Study the drawing (mm; zero at the part's minimum x, y, z) and answer. A direction names the side the tool comes from. Give positions to 0.01 mm unless a question says otherwise; leave off trailing zeros. Write each loop counter-clockwise with the first axis right and the second up, starting at its lowest first coordinate (ties: lowest second). Pieces come first, ordered by that corner, then holes. Notation, with made-up numbers: M 64.5,46 L 99.5,46 A14 cw 99.5,62 Z; hole C 77.5,31 d1. An arc over 180 degrees is marked long. Use a Markdown table: item, result. Add a question column.
Item 1: For the marked faces 1, 2, 3, 4 and 5, determine the directions among +Z, -Z, +X, -X, +Y, -Y from which every point of the face is accessible in a straight line to the end or side of a thin tool.
Item 2: Given P1, Ø7.5, axis at x = 6.35, y = 6.35, coming from the +Z side; P2, Ø3, axis at x = 7.5, z = 15.5, coming from the +Y side; P3, Ø1.5, axis at y = 4, z = 35.5, coming from the -X side; P4, Ø5, axis at x = 6, z = 9.5, coming from the -Y side, each flat-ended and moving along its own axis, determine where each tip first touches the part or whether it passes through.
Item 3: A cutting plane is placed at C-C on z = 29. Determine the outline of the cut face in (x, y), then the cut area to 3 significant figures.
Item 4: A cutting plane is placed at A-A on y = 6.35. Determine the outline of the cut face in (x, z) (3 decimals).
Item 5: A cutting plane is placed at B-B on x = 6.35. Determine the outline of the cut face in (y, z) (3 decimals), then the cut area to 3 significant figures.
Item 6: Consider probe 1 along Y at (x, z) = (6.35, 3) (3 decimals); probe 2 along X at (y, z) = (6.5, 15.5); probe 3 along Z at (x, y) = (4.75, 6.75) (3 decimals). Determine where each line is inside the solid, lowest interval first. Write a range as [from, to].
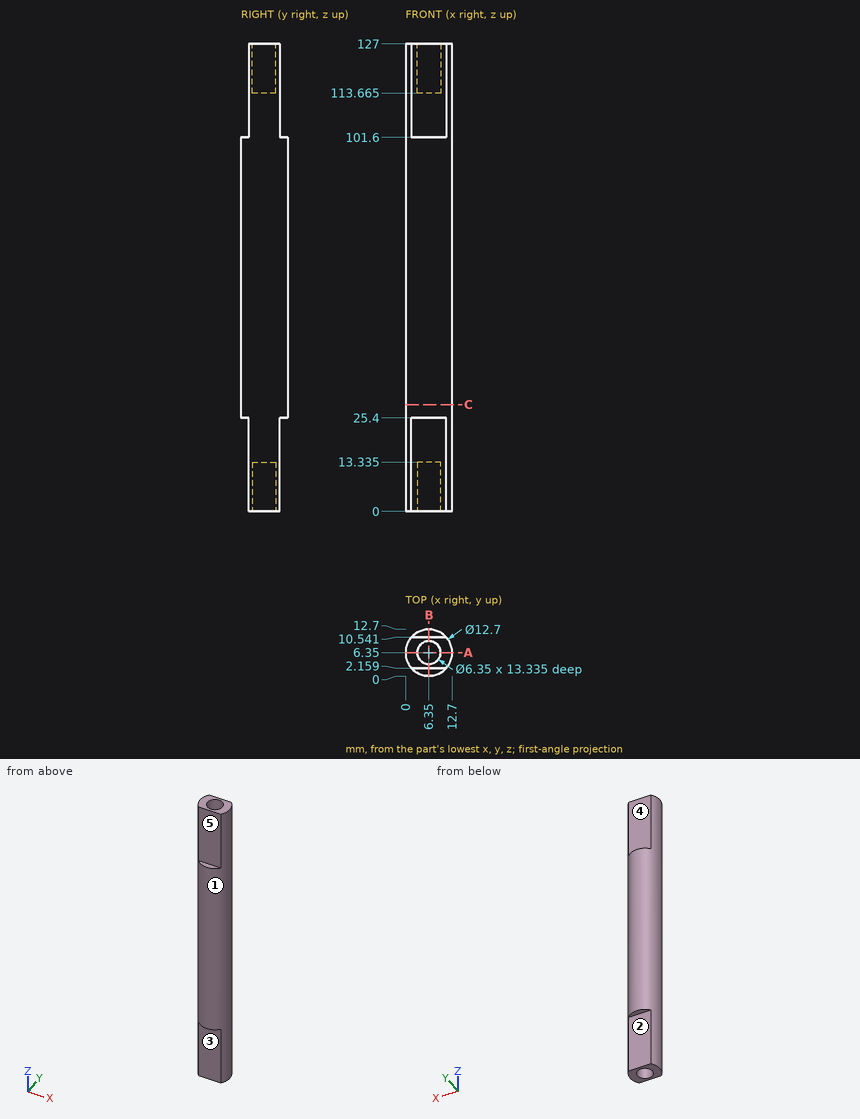
Filled in:
| question | item | result |
|---|---|---|
| 1 | face 1 | +Z, -Z |
| 1 | face 2 | -Z, +X, -X, +Y |
| 1 | face 3 | -Z, +X, -X, -Y |
| 1 | face 4 | +Z, +X, -X, +Y |
| 1 | face 5 | +Z, +X, -X, -Y |
| 2 | P1 | z = 127 |
| 2 | P2 | y = 10.54 |
| 2 | P3 | x = 0.2 |
| 2 | P4 | y = 2.16 |
| 3 | outline | C 6.35,6.35 d12.7 |
| 3 | area | 127 mm² |
| 4 | outline | M 0,0 L 3.175,0 L 3.175,13.335 L 9.525,13.335 L 9.525,0 L 12.7,0 L 12.7,127 L 9.525,127 L 9.525,113.665 L 3.175,113.665 L 3.175,127 L 0,127 Z |
| 5 | outline | M 0,25.4 L 2.159,25.4 L 2.159,0 L 3.175,0 L 3.175,13.335 L 9.525,13.335 L 9.525,0 L 10.541,0 L 10.541,25.4 L 12.7,25.4 L 12.7,101.6 L 10.541,101.6 L 10.541,127 L 9.525,127 L 9.525,113.665 L 3.175,113.665 L 3.175,127 L 2.159,127 L 2.159,101.6 L 0,101.6 Z |
| 5 | area | 1,220 mm² |
| 6 | probe 1 | [2.159, 3.175], [9.525, 10.541] |
| 6 | probe 2 | [0, 12.7] |
| 6 | probe 3 | [13.335, 113.665] |
